Could you check a few things on this drawing? It's one solid part, dimensions in mm from its lowest x, y, z. A direction names the side the tool comes from. Coordinates: 2 decimals unless noted, no trailing zeros. Loops run counter-clockwise (first coordinate to the right, second up) from the corner with the lowest first, then second, coordinate; pieces in that order, holes last. Notation, with made-up numbers: M -14,57 L -4,57 A5 ccw -4,63 Z; hole C 40,75 d8. An arc over 180 degrees is marked long. Answer as a JSON object with one key per item and string values. Group by question number.
Item 1: I'm going to push flat-ended pins straight in: pin 1 Ø3 at (x, y) = (7.5, 1.5) entering from +Z; pin 2 Ø1.5 at (y, z) = (1, 1.5) entering from +X. Where does each tip first touch, or does it pass through?
Item 2: We'd pull the mould along X, two halves only. Please class the marked faces 6, 7, 8 and 9: +X half, -X half, draft (parallel to the pull), parting line (faces both ways), or undercut.
Item 3: Which directions (+Z, -Z, +X, -X, +Y, -Y) give clear straight access to the entire face, cutting with the end or side of a thin tool? Please do the marked faces 1, 2, 3, 4 and 5.
Item 4: Suppose I cut it at A-A (x = 0.5). Write out the boundary of the cut face in (y, z).
Item 5: Suppose I cut it at D-D (x = 3.25). Write out the boundary of the cut face in (y, z), then the cut area to 3 significant figures.
Item 6: Suppose I cut it at B-B (y = 7.75). Write out the boundary of the cut face in (x, z).
Item 7: If I drill on line 1 (Z direction, x = 2.5, y = 2.5); line 2 (Y direction, x = 0.75, z = 1.05) (1 decimal); line 3 (X direction, y = 7.25, z = 1.35) (1 decimal), over which ranges is the centre line in solid material (lowest first)?
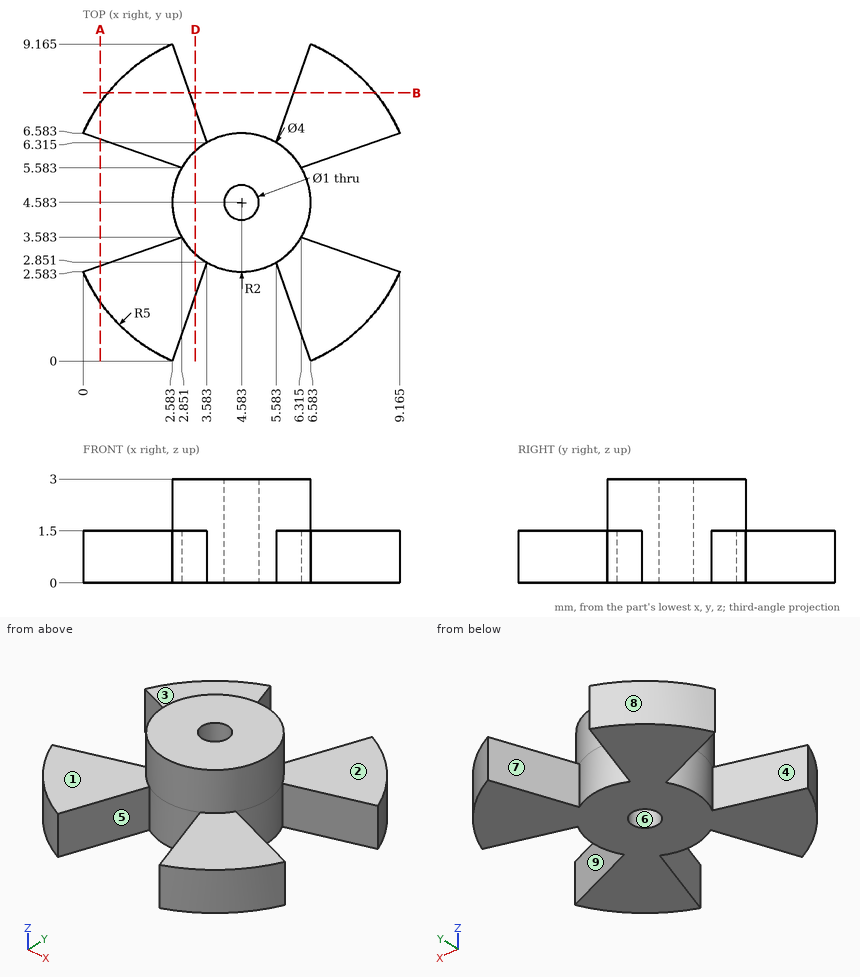
From the geometry:
{
 "1": {"pin 1": "z = 1.5", "pin 2": "x = 8.7"},
 "2": {"face 6": "undercut", "face 7": "undercut", "face 8": "-X half", "face 9": "+X half"},
 "3": {"face 1": "+Z, -X, -Y", "face 2": "+Z, +X, +Y", "face 3": "+Z, -X, +Y", "face 4": "+Z, -Z, -X", "face 5": "+Z, -Z, -Y"},
 "4": {"outline": "M 1.7,0 L 2.76,0 L 2.76,1.5 L 1.7,1.5 Z; M 6.41,0 L 7.47,0 L 7.47,1.5 L 6.41,1.5 Z"},
 "5": {"outline": "M 1.9,0 L 7.26,0 L 7.26,1.5 L 6.07,1.5 L 6.07,3 L 3.09,3 L 3.09,1.5 L 1.9,1.5 Z", "area": "12.5 mm2"},
 "6": {"outline": "M 0.71,0 L 3.08,0 L 3.08,1.5 L 0.71,1.5 Z; M 6.09,0 L 8.45,0 L 8.45,1.5 L 6.09,1.5 Z"},
 "7": {"line 1": "0 to 1.5", "line 2": "1.4 to 2.8, 6.3 to 7.8", "line 3": "0.4 to 3.3, 5.9 to 8.8"}
}
